```python
from build123d import *

# Parameters (mm, degrees)
CROQUIS1_W                   = 7.6
CROQUIS1_H                   = 5.8
SALIENTE_EXTRUIR1_DEPTH      = 3.2
CROQUIS2_W                   = 5.7
CROQUIS2_H                   = 0.9
SALIENTE_EXTRUIR2_DEPTH      = 8.2
REDONDEO2_R                  = 0.5
REDONDEO3_R                  = 0.5
CROQUIS3_W                   = 1
CROQUIS3_H                   = 5.8
CORTAR_EXTRUIR1_DEPTH        = 1
SALIENTE_EXTRUIR3_DEPTH      = 4.4
SALIENTE_EXTRUIR3_DEPTH_BACK = 10
CROQUIS4_W                   = 0.6
CROQUIS4_H                   = 0.6


with BuildPart() as part:
    # Croquis1 → Saliente-Extruir1 (new body)
    with BuildSketch(Plane(origin=(0, 0, 0), x_dir=(1, 0, 0), z_dir=(0, 1, 0))):
        Rectangle(CROQUIS1_W, CROQUIS1_H)
    extrude(amount=SALIENTE_EXTRUIR1_DEPTH)

    # Croquis2 → Saliente-Extruir2 (add)
    with BuildSketch(Plane(origin=(0, 3.2, 0), x_dir=(1, 0, 0), z_dir=(0, 1, 0))):
        with Locations((0, 2.45)):
            Rectangle(CROQUIS2_W, CROQUIS2_H)
    extrude(amount=SALIENTE_EXTRUIR2_DEPTH)

    # Redondeo2
    redondeo2_edges = [part.edges().sort_by_distance(p)[0] for p in [
        (2.85, 11.4, -2.45),
    ]]
    fillet(redondeo2_edges, radius=REDONDEO2_R)

    # Redondeo3
    redondeo3_edges = [part.edges().sort_by_distance(p)[0] for p in [
        (-2.85, 11.4, -2.45),
    ]]
    fillet(redondeo3_edges, radius=REDONDEO3_R)

    # Croquis3 → Cortar-Extruir1 (cut)
    with BuildSketch(Plane.XZ):
        with Locations((-2.5, 0)):
            Rectangle(CROQUIS3_W, CROQUIS3_H)
        Rectangle(CROQUIS3_W, CROQUIS3_H)
        with Locations((2.5, 0)):
            Rectangle(CROQUIS3_W, CROQUIS3_H)
    extrude(amount=-CORTAR_EXTRUIR1_DEPTH, mode=Mode.SUBTRACT)

    # Croquis4 → Saliente-Extruir3 (add, two sides: drawn at the far end of the back side and taken through both)
    with BuildSketch(Plane.XZ.offset(-1).offset(-SALIENTE_EXTRUIR3_DEPTH_BACK)):
        with Locations((-2.5, -0.5)):
            Rectangle(CROQUIS4_W, CROQUIS4_H)
        with Locations((0, -0.5)):
            Rectangle(CROQUIS4_W, CROQUIS4_H)
        with Locations((2.5, -0.5)):
            Rectangle(CROQUIS4_W, CROQUIS4_H)
    extrude(amount=SALIENTE_EXTRUIR3_DEPTH + SALIENTE_EXTRUIR3_DEPTH_BACK)


solid = part.part
```
Design review of the part built by this model. Coordinates are the model's own, in mm. A direction names the side the tool comes from. Give positions to 0.01 mm unless a question says otherwise; leave off trailing zeros. Order: outer loops, then holes, each group sorted by start corner. A loop starts at its lowest first (then second) coordinate and runs counter-clockwise, first axis right, second up. Notation, with made-up numbers: M 11,20.25 L 29,20.25 A17 ccw 29,41.25 Z; hole C 22,-36 d4. An arc over 180 degrees is marked long. One line per question, with ' | ' between items. Start each with the question number.
Q1. We need section C-C (y = -1.5). Write out the cut boundary in (x, z).
Q2. For pin 1 Ø3 at (x, y) = (1, 4) entering from +Z; pin 2 Ø0.7 at (x, y) = (-2.5, -1.5) entering from +Z; pin 3 Ø0.8 at (x, z) = (2.5, 0.5) entering from -Y; pin 4 Ø3 at (y, z) = (7.5, 0.5) entering from +X, all flat-tipped, find the tip position at first contact; note any pin that passes through.
Q3. We need section B-B (z = 1.75). Write out the cut boundary in (x, y), plus the area to 3 significant figures.
Q4. We need section D-D (x = -1.75). Write out the cut boundary in (y, z).
Q5. The part is to be moulded in two halves that separate along X. For faces 1 (the face through (-2, 0.5, 0)), 2 (the face through (0, 2, 2.9)), 3 (the face through (3, 0.5, 0)), 4 (the face through (2.85, 7, -2.4)), say which applies: +X half, -X half, draft (parallel to the pull), parting line (faces both ways), or undercut.
Q6. For L1, parallel to X at y = 0.5, z = 1.95; L2, parallel to X at y = 10.75, z = -0.7; L3, parallel to Z at x = 0, y = 6, list the stretches that pass through material, from the lowest coordinate up. Write a range as [from, to].
Q7. We need section A-A (y = 7). Write out the cut boundary in (x, z), plus the area to 3 significant figures.
Q8. Machinability: for faces 5 (the face through (-2.85, 7, -2.4)), 6 (the face through (-3, 0.5, 0)), 7 (the face through (0, 7, -2)), which of the approach directions +Z, -Z, +X, -X, +Y, -Y give a long, thin tool a straight path to every point of the face, cutting with its end or side? Answer none if there is none.
Returned:
1) outline: M -2.8,-0.8 L -2.2,-0.8 L -2.2,-0.2 L -2.8,-0.2 Z; M -0.3,-0.8 L 0.3,-0.8 L 0.3,-0.2 L -0.3,-0.2 Z; M 2.2,-0.8 L 2.8,-0.8 L 2.8,-0.2 L 2.2,-0.2 Z
2) pin 1: z = 2.9 | pin 2: z = -0.2 | pin 3: y = 1 | pin 4: x = 2.8
3) outline: M -3.8,0 L -3,0 L -3,1 L -2,1 L -2,0 L -0.5,0 L -0.5,1 L 0.5,1 L 0.5,0 L 2,0 L 2,1 L 3,1 L 3,0 L 3.8,0 L 3.8,3.2 L -3.8,3.2 Z | area: 21.3 mm2
4) outline: M 0,-2.9 L 11.4,-2.9 L 11.4,-2 L 3.2,-2 L 3.2,2.9 L 0,2.9 Z
5) face 1: undercut | face 2: draft | face 3: undercut | face 4: +X half
6) L1: [-3.8, -3], [-2, -0.5], [0.5, 2], [3, 3.8] | L2: [-2.8, -2.2], [-0.3, 0.3], [2.2, 2.8] | L3: [-2.9, -2], [-0.8, -0.2]
7) outline: M -2.85,-2.9 L 2.85,-2.9 L 2.85,-2 L -2.85,-2 Z; M -2.8,-0.8 L -2.2,-0.8 L -2.2,-0.2 L -2.8,-0.2 Z; M -0.3,-0.8 L 0.3,-0.8 L 0.3,-0.2 L -0.3,-0.2 Z; M 2.2,-0.8 L 2.8,-0.8 L 2.8,-0.2 L 2.2,-0.2 Z | area: 6.21 mm2
8) face 5: +Z, -Z, -X, +Y | face 6: +Z, -Z, -Y | face 7: +X, -X, +Y
